Autodesk Inventor part; units mm, degrees
ref_plane "YZ Plane" through (0, 0, 0) normal (1, 0, 0) x (0, 1, 0)
ref_plane "XZ Plane" through (0, 0, 0) normal (0, 1, 0) x (-1, 0, 0)
ref_plane "XY Plane" through (0, 0, 0) normal (0, 0, 1) x (1, 0, 0)
sketch "Sketch1" plane through (0, 0, 0) normal (0, 0, 1) x (1, 0, 0)
  line L0 (-52.5, 5) -> (-47.5, 5)
  line L1 (-47.5, 5) -> (-47.5, 56)
  line L2 (-47.5, 56) -> (47.5, 56)
  line L3 (47.5, 56) -> (47.5, 5)
  line L4 (47.5, 5) -> (52.5, 5)
  line L5 (-42.5, 0) -> (-42.5, 51)
  line L6 (-42.5, 51) -> (42.5, 51)
  line L7 (42.5, 51) -> (42.5, 0)
  line L8 (0, 0) -> (0, -25.7238) construction
  line L9 (52.5, 0) -> (52.5, 5)
  line L10 (-52.5, 0) -> (-52.5, 5)
  line L11 (-52.5, 0) -> (-42.5, 0)
  line L12 (42.5, 0) -> (52.5, 0)
  line L13 (-32.5, 56) -> (-12.5, 56)
  line L14 (-12.5, 56) -> (-12.5, 51)
  line L15 (-12.5, 51) -> (-32.5, 51)
  line L16 (-32.5, 51) -> (-32.5, 56)
  line L17 (12.5, 56) -> (32.5, 56)
  line L18 (32.5, 56) -> (32.5, 51)
  line L19 (32.5, 51) -> (12.5, 51)
  line L20 (12.5, 51) -> (12.5, 56)
  line L21 (-32.5, 56) -> (-12.5, 56)
  line L22 (-12.5, 56) -> (-12.5, 11)
  line L23 (-12.5, 11) -> (-32.5, 11)
  line L24 (-32.5, 11) -> (-32.5, 56)
  line L25 (12.5, 56) -> (32.5, 56)
  line L26 (32.5, 56) -> (32.5, 11)
  line L27 (32.5, 11) -> (12.5, 11)
  line L28 (12.5, 11) -> (12.5, 56)
  point P0 (32.5, 56)
  point P1 (-32.5, 51)
  point P2 (-12.5, 56)
  point P3 (32.5, 56)
  point P4 (-32.5, 56)
  dimension "d1" = 5
  dimension "d2" = 5
  dimension "d3" = 5
  dimension "d5" = 85
  dimension "d6" = 51
  dimension "d8" = 5
  dimension "d18" = 105
  dimension "d19" = 20
  dimension "d20" = 25
  dimension "d21" = 45
extrude "Extrusion1" add sketch "Sketch1" along normal mid plane 20 contours L0 L1 L2 L16 L6 L5 L11 L10 | L2 L14 L6 L16 | L2 L20 L6 L14 | L2 L18 L6 L20 | L2 L3 L4 L9 L12 L7 L6 L18
sketch "Sketch2" plane through (-52.5, 0, 10) normal (0, -1, 0) x (1, 0, 0)
  circle A0 centre (2.5, -10) radius 1.25
  circle A1 centre (102.5, -10) radius 1.25
  line L0 (52.5, -10) -> (52.5, 0) construction
  line L1 (10, 0) -> (95, 0) construction
  circle A2 centre (2.5, -10) radius 2.25
  circle A3 centre (102.5, -10) radius 2.25
  dimension "d11" = 2.5
  dimension "d12" = 100
  dimension "d15" = 4.5
extrude "Extrusion2" cut sketch "Sketch2" against normal through all contours A0 | A1
extrude "Extrusion4" add sketch "Sketch1" along normal blind 28 from surface at 10 contours L2 L14 L6 L16 | L2 L18 L6 L20
extrude "Extrusion5" add sketch "Sketch1" along normal blind 5 from surface at 38 contours L2 L14 L6 L16 | L6 L22 L23 L24 | L2 L18 L6 L20 | L6 L26 L27 L28
mirror "Mirror1" about plane through (0, 0, 0) normal (0, 0, 1) of "Extrusion5", "Extrusion4"
sketch "Sketch3" plane through (42.5, 51, -10) normal (0, -1, 0) x (1, 0, 0)
  line L0 (-55, 20) -> (-30, 20)
  line L1 (-36.5, 0) -> (-48.5, 0)
  line L2 (-48.5, 0) -> (-48.5, 20)
  line L3 (-48.5, 20) -> (-36.5, 20)
  line L4 (-36.5, 20) -> (-36.5, 0)
  line L5 (-36.5, 0) -> (-48.5, 20) construction
  line L6 (-48.5, 0) -> (-36.5, 20) construction
  point P0 (-42.5, 10)
  dimension "d26" = 12
extrude "Extrusion6" add sketch "Sketch3" along normal blind 5
equation "\"d1\" = d8"
equation "\"d2\" = d8"
equation "\"d3\" = d8"
properties part number "battery_fix"
Source: CAD feature listing. Evaluate the final solid. Frame: model axes, mm. A direction names the side the tool comes from. Give positions to 0.01 mm unless a question says otherwise; leave off trailing zeros. Order: outer loops, then holes, each group sorted by start corner. A loop starts at its lowest first (then second) coordinate and runs counter-clockwise, first axis right, second up. Notation, with made-up numbers: (-26.5, -28) -> (-20.5, -28) arc R31 cw to (-20.5, 9) -> close; hole circle Ø11 at (19, 58). An arc over 180 degrees is marked (long way). Write item = value, one per line.
Item 1: Section query B-B (z = 14). Output: boundary loops of the cut face in (x, y).
Check result:
outline = (-32.5, 51) -> (-12.5, 51) -> (-12.5, 56) -> (-32.5, 56) -> close; (12.5, 51) -> (32.5, 51) -> (32.5, 56) -> (12.5, 56) -> close
Item 2: Section query D-D (x = 17.5). Output: boundary loops of the cut face in (y, z), then the cut area to 3 significant figures.
Check result:
outline = (11, -43) -> (56, -43) -> (56, 43) -> (11, 43) -> (11, 38) -> (51, 38) -> (51, -38) -> (11, -38) -> close
area = 830 mm²
Item 3: Ray query, probe 1 along Z at (x, y) = (50, 2.1); probe 2 along Z at (x, y) = (-25, 29); probe 3 along X at (y, z) = (48.5, -7). Return the intervals inside material, ascending.
Check result:
probe_1 = -10 to -1.25, 1.25 to 10
probe_2 = -43 to -38, 38 to 43
probe_3 = -47.5 to -42.5, -6 to 6, 42.5 to 47.5
Item 4: Section query C-C (y = 23). Output: boundary loops of the cut face in (x, z), then the cut area to 3 significant figures.
Check result:
outline = (-47.5, -10) -> (-42.5, -10) -> (-42.5, 10) -> (-47.5, 10) -> close; (-32.5, -43) -> (-12.5, -43) -> (-12.5, -38) -> (-32.5, -38) -> close; (-32.5, 38) -> (-12.5, 38) -> (-12.5, 43) -> (-32.5, 43) -> close; (12.5, -43) -> (32.5, -43) -> (32.5, -38) -> (12.5, -38) -> close; (12.5, 38) -> (32.5, 38) -> (32.5, 43) -> (12.5, 43) -> close; (42.5, -10) -> (47.5, -10) -> (47.5, 10) -> (42.5, 10) -> close
area = 600 mm²
Item 5: Section query A-A (x = -50). Output: boundary loops of the cut face in (y, z).
Check result:
outline = (0, -10) -> (5, -10) -> (5, -1.25) -> (0, -1.25) -> close; (0, 1.25) -> (5, 1.25) -> (5, 10) -> (0, 10) -> close
Item 6: Set-up query: faces 4 (the face through (0, 46, 0)), 5 (the face through (12.5, 42, 39)), 6 (the face through (32.5, 42, 39)). Return all of +Z, -Z, +X, -X, +Y, -Y with unobstructed straight access to the full face (end or side cutting, diameter ignored); none if empty.
Check result:
face_4 = +Z, -Z, -Y
face_5 = +Z, +Y, -Y
face_6 = +Z, +X, +Y, -Y
Item 7: Mould query, pull axis Z, two halves, no side actions, for faces 1 (the face through (0, 52, 10)), 2 (the face through (22, 31, 38)), 3 (the face through (52.5, 2, 0)). Classes: +Z half, -Z half, draft (parallel to the pull), parting line (faces both ways), or undercut.
Check result:
face_1 = +Z half
face_2 = undercut
face_3 = draft
Item 8: Contact query for flat-ended pins moving along their axis: pin 1 (10 mm diameter, centred on y = 27, z = -32.5, fed in from -X); pin 2 (5 mm diameter, centred on x = -11, z = -23, fed in from -Y); pin 3 (16 mm diameter, centred on x = 46.5, y = 36, fed in from +Z); pin 4 (4 mm diameter, centred on x = 18.5, z = 40, fed in from -Y). Output: stop coordinate, or through.
Check result:
pin_1 = through
pin_2 = 51
pin_3 = 10
pin_4 = 11
